Input: dimensioned drawing with shaded views. Units: mm. Origin: part minimum x, y, z. Round coordinates to 2 decimals unless told otherwise and drop trailing zeros. Order: outer loops, then holes, each group sorted by start corner. A loop starts at its lowest first (then second) coordinate and runs counter-clockwise, first axis right, second up. Notation, with made-up numbers: (-17, 55.25) - (20, 55.25) arc R22 ccw to (20, 87.25) - close; hole circle Ø9 at (54, 51). An arc over 180 degrees is marked (long way). Return JSON: item names as keys, results as strings. Group by question number.
1) Section C-C, the plane y = 0.4. Give the number of separate pieces and of enclosed holes in the cut face, plus the area to 3 significant figures.
2) Section A-A, the plane z = 29. Return loops of the section in (x, y).
3) Ray query, line 1 (X direction, y = 0.5, z = 2); line 2 (X direction, y = 0.6, z = 25). Return the intervals inside material, ascending. Write a range as from..to.
4) Section B-B, the plane x = 17.5. Return loops of the section in (y, z).
5) Contact query for flat-ended pins moving along their axis: P1, Ø13.5, axis at x = 25, z = 25, coming from the -Y side; P2, Ø4, axis at x = 2, z = 48, coming from the +Y side. Output: stop coordinate, or through.
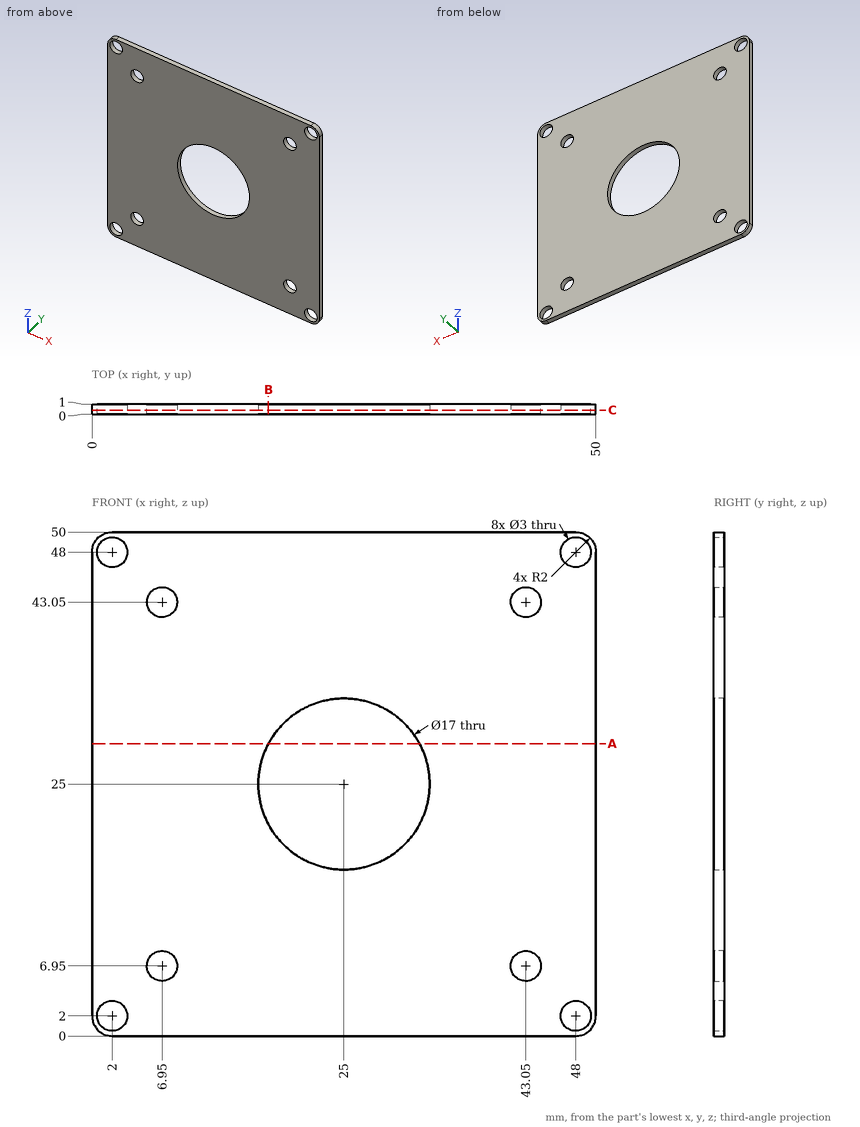
Geometry check:
{
 "1": {"separate pieces": "1", "enclosed holes": "9", "area": "2,210 mm2"},
 "2": {"outline": "(0, 0) - (17.5, 0) - (17.5, 1) - (0, 1) - close; (32.5, 0) - (50, 0) - (50, 1) - (32.5, 1) - close"},
 "3": {"line 1": "0..0.5, 3.5..46.5, 49.5..50", "line 2": "0..16.5, 33.5..50"},
 "4": {"outline": "(0, 0) - (1, 0) - (1, 21) - (0, 21) - close; (0, 29) - (1, 29) - (1, 50) - (0, 50) - close"},
 "5": {"P1": "through", "P2": "y = 1"}
}
